Geometry: final body of the model. Coordinates: model frame, mm. Coordinates: 2 decimals unless noted, no trailing zeros. Order: outer loops, then holes, each group sorted by start corner. A loop starts at its lowest first (then second) coordinate and runs counter-clockwise, first axis right, second up. Notation, with made-up numbers: (0, 39) - (53, 39) arc R31 cw to (53, 77) - close; hole circle Ø6 at (80.25, 12.25). An arc over 180 degrees is marked (long way). Use one line per item in the form item = value. Start each with the question number.
Autodesk Inventor part; units mm, degrees
ref_plane "Work Plane1" through (15.24, 0, -4.7625) normal (0, 0, -1) x (-1, 0, 0)
ref_plane "YZ Plane" through (0, 0, 0) normal (1, 0, 0) x (0, 1, 0)
ref_plane "XZ Plane" through (0, 0, 0) normal (0, 1, 0) x (-1, 0, 0)
sketch "Sketch1" plane through (0, 0, 0) normal (0, 1, 0) x (-1, 0, 0)
  line L0 (0, 0) -> (0, -9.525)
  line L1 (-15.24, 4.2545) -> (-15.24, -13.7795)
  line L2 (0, 0) -> (-15.24, 4.2545)
  line L3 (0, -9.525) -> (-15.24, -13.7795)
  line L4 (-15.24, 4.2545) -> (-19.05, 4.2545)
  line L5 (-19.05, 4.2545) -> (-19.05, 2.9845)
  line L6 (-19.05, 2.9845) -> (-15.24, 2.9845)
  line L7 (-15.24, 2.9845) -> (-15.24, 4.2545)
  line L8 (-15.24, -13.7795) -> (-19.05, -13.7795)
  line L9 (-19.05, -13.7795) -> (-19.05, -12.5095)
  line L10 (-19.05, -12.5095) -> (-15.24, -12.5095)
  line L11 (-15.24, -12.5095) -> (-15.24, -13.7795)
  line L12 (0, 0) -> (0, 3.175)
  line L13 (-15.24, 4.2545) -> (-15.24, 7.4295)
  line L14 (0, -9.525) -> (0, -12.7)
  line L15 (-15.24, -13.7795) -> (-15.24, -16.9545)
  line L16 (-15.24, -16.9545) -> (0, -12.7)
  line L17 (0, 3.175) -> (-15.24, 7.4295)
  line L18 (-15.24, 7.4295) -> (-34.29, 7.4295)
  line L19 (-19.05, 4.2545) -> (-34.29, 4.2545)
  line L20 (-34.29, 4.2545) -> (-34.29, 7.4295)
  line L21 (-15.24, -16.9545) -> (-34.29, -16.9545)
  line L22 (-34.29, -16.9545) -> (-34.29, -13.7795)
  line L23 (-34.29, -13.7795) -> (-19.05, -13.7795)
  line L24 (-34.29, 7.4295) -> (-37.465, 7.4295)
  line L25 (-37.465, 7.4295) -> (-37.465, -17.5895)
  line L26 (-37.465, -17.5895) -> (-34.29, -17.5895)
  line L27 (-34.29, -17.5895) -> (-34.29, 7.4295)
  line L28 (-15.24, -13.7795) -> (-34.29, -13.7795)
  line L29 (-34.29, -13.7795) -> (-34.29, 4.2545)
  line L30 (-34.29, 4.2545) -> (-15.24, 4.2545)
  line L31 (-15.24, 4.2545) -> (-15.24, -13.7795)
  line L32 (-15.24, 4.2545) -> (-34.29, 4.2545)
  line L33 (-34.29, 4.2545) -> (-34.29, 7.4295)
  line L34 (-34.29, 7.4295) -> (-15.24, 7.4295)
  line L35 (-15.24, 7.4295) -> (-15.24, 4.2545)
  line L36 (-15.24, -7.5565) -> (-22.86, -7.5565)
  line L37 (-22.86, -7.5565) -> (-22.86, -1.9685)
  line L38 (-22.86, -1.9685) -> (-15.24, -1.9685)
  line L39 (-15.24, -1.9685) -> (-15.24, -7.5565)
  dimension "d0" = 9.525
  dimension "d1" = 15.24
  dimension "d2" = 18.034
  dimension "d3" = 4.2545
  dimension "d4" = 3.81
  dimension "d5" = 1.27
  dimension "d6" = 3.81
  dimension "d7" = 1.27
  dimension "d8" = 3.175
  dimension "d9" = 3.175
  dimension "d10" = 3.175
  dimension "d11" = 3.175
  dimension "d12" = 19.05
  dimension "d13" = 3.175
  dimension "d30" = 7.62
  dimension "d31" = 5.588
  dimension "d32" = 6.223
extrude "Extrusion6" add sketch "Sketch1" along normal blind 5.588 contours L0 L3 L1 L2 | L1 L36 L37 L38
sketch "Sketch5" plane through (0, 5.588, 0) normal (0, 1, 0) x (1, 0, 0)
  circle A0 centre (8.636, 4.7625) radius 1.5875
  line L0 (0, 9.525) -> (0, 0)
  dimension "d35" = 3.175
  dimension "d36" = 8.636
extrude "Extrusion7" cut sketch "Sketch5" against normal blind 5.588
sketch "Sketch6" plane through (15.24, 0, 4.2545) normal (1, 0, 0) x (0, 0, -1)
  line L0 (6.223, 0) -> (6.223, 5.588)
  line L1 (0, 5.588) -> (6.223, 5.588)
  line L2 (0, 0) -> (0, 5.588)
  line L3 (0, 0) -> (6.223, 0)
  line L4 (11.811, 5.588) -> (11.811, 0)
  line L5 (11.811, 0) -> (18.034, 0)
  line L6 (18.034, 0) -> (18.034, 5.588)
  line L7 (11.811, 5.588) -> (18.034, 5.588)
  circle A0 centre (1.863, 2.794) radius 0.381
  circle A1 centre (4.4524, 2.794) radius 0.381
  line L8 (6.223, 5.588) -> (11.811, 5.588)
  line L9 (9.017, 5.588) -> (9.017, 8.4963)
  circle A2 centre (16.171, 2.794) radius 0.381
  circle A3 centre (13.5816, 2.794) radius 0.381
  point P0 (4.2545, 0)
  dimension "d39" = 0.762
  dimension "d40" = 0.762
extrude "Extrusion8" add sketch "Sketch6" along normal blind 6.35 contours A0 | A1 | A2 | A3
ref_plane "Work Plane1" through (15.24, 0, -4.7625) normal (0, 0, -1) x (-1, 0, 0)
equation "\"d3\" = -0.5 * d0 + 0.5 * d2"
equation "\"d32\" = -0.5 * d31 + 0.5 * d2"
properties part number "photoTransistor" material "ABS Plastic"
(1) Cut plane A-A on x = 20.25. Return the cut outline in (y, z), plus the area to 3 significant figures.
(2) Draft query along Z for faces 1 (the flat face through (12, 0, -5)), 2 (the cylindrical face through (7.05, 2.83, -4.83)), 3 (the flat face through (7.513, 2.755, 2.097)). Return one class per face: released by +Z, released by -Z, zero draft, split by the parting line, or undercut.
(3) Material intervals for L1, parallel to Z at x = 8.75, y = 2; L2, parallel to Z at x = 8, y = 1; L3, parallel to Z at x = 16.75, y = 3.9, sorted ascending. Write a range as from..to.
(4) Cut plane D-D on x = 6. Return the cut outline in (y, z) (3 decimals).
(5) Contact query for flat-ended pins moving along their axis: pin 1 Ø1.7 at (x, y) = (18, 2) entering from +Z; pin 2 Ø0.6 at (y, z) = (2.5, 2.5) entering from +X; pin 3 Ø1 at (x, y) = (8, 3.5) entering from -Z. Output: stop coordinate, or through.
(6) Cut plane B-B on y = 1.15. Return the cut outline in (x, z) (1 decimal).
(7) Cut plane C-C on z = -0.25. Return the cut outline in (x, y).
Check sheet entries:
q1.outline = (0, -7.56) - (5.59, -7.56) - (5.59, -1.97) - (0, -1.97) - close; circle Ø0.76 at (2.79, -11.92); circle Ø0.76 at (2.79, -9.33); circle Ø0.76 at (2.79, -0.2); circle Ø0.76 at (2.79, 2.39)
q1.area = 33.0 mm^2
q2.face_1 = zero draft
q2.face_2 = undercut
q2.face_3 = released by +Z
q3.L1 = -11.97..-6.35, -3.18..2.44
q3.L2 = -11.76..-6.22, -3.31..2.23
q3.L3 = -7.56..-1.97
q4.outline = (0, -11.2) - (5.588, -11.2) - (5.588, 1.675) - (0, 1.675) - close
q5.pin_1 = 2.77
q5.pin_2 = 21.59
q5.pin_3 = -11.9
q6.outline = (0, -9.5) - (15.2, -13.8) - (15.2, -7.6) - (22.9, -7.6) - (22.9, -2) - (15.2, -2) - (15.2, 4.3) - (0, 0) - close; hole circle Ø3.2 at (8.6, -4.8)
q7.outline = (0, 0) - (15.24, 0) - (15.24, 2.42) - (21.59, 2.42) - (21.59, 3.17) - (15.24, 3.17) - (15.24, 5.59) - (0, 5.59) - close
